Read the model definition and answer for the solid it produces. Units are mm, in the model's axes. A direction names the side the tool comes from. Give positions to 0.01 mm unless a question says otherwise; leave off trailing zeros. Order: outer loops, then holes, each group sorted by start corner. A loop starts at its lowest first (then second) coordinate and runs counter-clockwise, first axis right, second up. Notation, with made-up numbers: (86.5, -14) - (90.5, -14) arc R21 cw to (90.5, 2) - close; hole circle Ø1 at (62.25, 5). An arc over 180 degrees is marked (long way). Use a Markdown table: item, result. Add a question column.
1. For a pull along Y with two mould halves and no side action, classify faces 4 (the flat face through (0, 0, 5)), 5 (the flat face through (-34, 5, 4)), 6 (the flat face through (-30, -14, 5)), 7 (the cylindrical face through (9.43, -5.6, 5.04)) as released by +Y, released by -Y, zero draft, split by the parting line, or undercut.
2. A cutting plane is placed at B-B on y = 2. Determine the outline of the cut face in (x, z), and give its area (3 significant figures).
3. Consider L1, parallel to Z at x = -35, y = -2; L2, parallel to Y at x = 4.5, z = 6; L3, parallel to X at y = 18.5, z = 5. Determine where each line is inside the solid, lowest interval first.
4. A cutting plane is placed at D-D on z = 5. State how many separate pieces and enclosed holes the cut face has, and give its area (3 significant figures).
5. A cutting plane is placed at A-A on x = -35. Determine the outline of the cut face in (y, z).
6. Which of the six approach directions +Z, -Z, +X, -X, +Y, -Y give full straight-line access (tool end or side, diameter ignored) to faces 1 (the cylindrical face through (-29.43, 13.66, 9.4)), 2 (the cylindrical face through (5.04, 5.57, 0.6)), 3 (the cylindrical face through (-29.43, 13.66, 0.6))?
7. Flat-ended cylindrical pins translate along their axes: P1, Ø6, axis at y = 1.5, z = 8.5, coming from the +X side; P2, Ø1.8, axis at y = 11, z = 4, coming from the -X side; P3, Ø1.8, axis at x = -35, z = 5, coming from the +Y side; P4, Ø1.8, axis at x = -33.5, z = 4, coming from the +Y side. Find the tip coordinate at first contact, or state that the pin passes through.
8. A cutting plane is placed at C-C on x = 5. Determine the outline of the cut face in (y, z), and give its area (3 significant figures).
```python
from build123d import *

# Parameters (mm, degrees)
BOSS_EXTRUDE1_DEPTH     = 10
FILLET1_R               = 2
CUT_EXTRUDE1_DEPTH      = 50.560569004
CUT_EXTRUDE1_DEPTH_BACK = 50.560569004
SKETCH2_R               = 1


with BuildPart() as part:
    # Sketch1 → Boss-Extrude1 (new body)
    with BuildSketch(Plane.XY):
        Polygon((10, 22.5), (-30, 22.5), (-30, 5), (-40, 5), (-40, -5), (-30, -5), (-30, -22.5), (10, -22.5), (10, -5), (0, -5), (0, 5), (10, 5), align=None)
    extrude(amount=BOSS_EXTRUDE1_DEPTH)

    # Fillet1
    fillet1_edges = [part.edges().sort_by_distance(p)[0] for p in [
        (-30, 13.75, 0),
        (-10, 22.5, 0),
        (-35, -5, 10),
        (10, 13.75, 0),
        (5, 5, 0),
        (0, 0, 0),
        (5, -5, 0),
        (10, -13.75, 0),
        (-10, -22.5, 0),
        (-30, -13.75, 0),
        (-35, -5, 0),
        (-40, 0, 0),
        (-35, 5, 0),
        (-30, -13.75, 10),
        (-30, 5, 5),
        (-30, 22.5, 5),
        (10, 22.5, 5),
        (-10, -22.5, 10),
        (10, 5, 5),
        (0, 5, 5),
        (0, -5, 5),
        (10, -5, 5),
        (10, -22.5, 5),
        (-30, -22.5, 5),
        (-30, -5, 5),
        (-40, -5, 5),
        (-40, 5, 5),
        (10, -13.75, 10),
        (5, -5, 10),
        (0, 0, 10),
        (5, 5, 10),
        (10, 13.75, 10),
        (-10, 22.5, 10),
        (-30, 13.75, 10),
        (-35, 5, 10),
        (-40, 0, 10),
    ]]
    fillet(fillet1_edges, radius=FILLET1_R)

    # Sketch2 → Cut-Extrude1 (cut, two sides: drawn at the far end of the back side and taken through both)
    with BuildSketch(Plane.XZ.offset(-5).offset(-CUT_EXTRUDE1_DEPTH_BACK)):
        with Locations(Location((5, 5, 0), (0, 0, 270))):
            Circle(SKETCH2_R)
        with Locations(Location((-35, 5, 0), (0, 0, 180))):
            Circle(SKETCH2_R)
    extrude(amount=CUT_EXTRUDE1_DEPTH + CUT_EXTRUDE1_DEPTH_BACK, mode=Mode.SUBTRACT)


solid = part.part
```
Output values:
| question | item | result |
|---|---|---|
| 1 | face 4 | undercut |
| 1 | face 5 | released by +Y |
| 1 | face 6 | zero draft |
| 1 | face 7 | undercut |
| 2 | outline | (-40, 2) arc R2 ccw to (-38, 0) - (-2, 0) arc R2 ccw to (0, 2) - (0, 8) arc R2 ccw to (-2, 10) - (-38, 10) arc R2 ccw to (-40, 8) - close; hole circle Ø2 at (-35, 5) |
| 2 | area | 393 mm² |
| 3 | L1 | 0 to 4, 6 to 10 |
| 3 | L2 | -22.5 to -5, 5 to 22.5 |
| 3 | L3 | -30 to 4, 6 to 10 |
| 4 | separate pieces | 4 |
| 4 | enclosed holes | 0 |
| 4 | area | 1,710 mm² |
| 5 | outline | (-5, 2) arc R2 ccw to (-3, 0) - (3, 0) arc R2 ccw to (5, 2) - (5, 4) - (-5, 4) - close; (-5, 6) - (5, 6) - (5, 8) arc R2 ccw to (3, 10) - (-3, 10) arc R2 ccw to (-5, 8) - close |
| 6 | face 1 | +Z, -X, +Y |
| 6 | face 2 | -Z, +X |
| 6 | face 3 | -Z, -X, +Y |
| 7 | P1 | x = 0.65 |
| 7 | P2 | x = -30 |
| 7 | P3 | through |
| 7 | P4 | y = 5 |
| 8 | outline | (-22.5, 2) arc R2 ccw to (-20.5, 0) - (-7, 0) arc R2 ccw to (-5, 2) - (-5, 4) - (-22.5, 4) - close; (-22.5, 6) - (-5, 6) - (-5, 8) arc R2 ccw to (-7, 10) - (-20.5, 10) arc R2 ccw to (-22.5, 8) - close; (5, 2) arc R2 ccw to (7, 0) - (20.5, 0) arc R2 ccw to (22.5, 2) - (22.5, 4) - (5, 4) - close; (5, 6) - (22.5, 6) - (22.5, 8) arc R2 ccw to (20.5, 10) - (7, 10) arc R2 ccw to (5, 8) - close |
| 8 | area | 273 mm² |
